The figure shows three views and two pictorial views of one solid part (mm, origin at its lowest corner). Answer the questions. Give positions to 0.01 mm unless a question says otherwise; leave off trailing zeros. Order: outer loops, then holes, each group sorted by start corner. A loop starts at its lowest first (then second) coordinate and runs counter-clockwise, first axis right, second up. Notation, with made-up numbers: (41, 51) - (88, 51) arc R12 ccw to (88, 67) - close; hole circle Ø2 at (62.25, -32). An arc over 180 degrees is marked (long way). Write item = value, one per line.
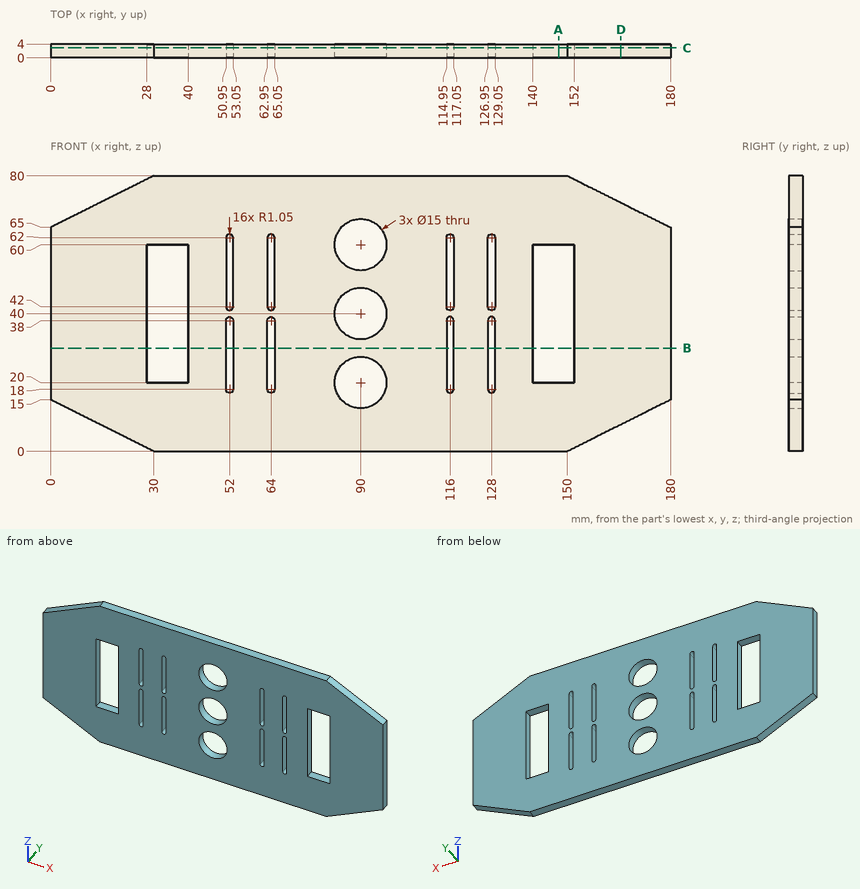
1. Section C-C (y = 2.85) is taken. Count the separate pieces of the cut face and the enclosed holes in it, and give its area (3 significant figures).
Recorded:
separate_pieces = 1
enclosed_holes = 13
area = 11,600 mm^2
2. Straight lines are drawn through the part: L1, parallel to X at y = 1.2, z = 40; L2, parallel to Z at x = 90, y = 1.85; L3, parallel to X at y = 1.35, z = 61.5. For each, find the intervals that lie inside material, in ascending order. Write a range as [from, to].
Recorded:
L1 = [0, 28], [40, 82.5], [97.5, 140], [152, 180]
L2 = [0, 12.5], [27.5, 32.5], [47.5, 52.5], [67.5, 80]
L3 = [0, 50.95], [53.05, 62.95], [65.05, 82.65], [97.35, 114.95], [117.05, 126.95], [129.05, 180]
3. Section B-B (z = 30) is taken. Determine the outline of the cut face in (x, y).
Recorded:
outline = (0, 0) - (28, 0) - (28, 4) - (0, 4) - close; (40, 0) - (50.95, 0) - (50.95, 4) - (40, 4) - close; (53.05, 0) - (62.95, 0) - (62.95, 4) - (53.05, 4) - close; (65.05, 0) - (114.95, 0) - (114.95, 4) - (65.05, 4) - close; (117.05, 0) - (126.95, 0) - (126.95, 4) - (117.05, 4) - close; (129.05, 0) - (140, 0) - (140, 4) - (129.05, 4) - close; (152, 0) - (180, 0) - (180, 4) - (152, 4) - close
4. Section A-A (x = 147.5) is taken. Determine the outline of the cut face in (y, z), and give its area (3 significant figures).
Recorded:
outline = (0, 0) - (4, 0) - (4, 20) - (0, 20) - close; (0, 60) - (4, 60) - (4, 80) - (0, 80) - close
area = 160 mm^2
5. Section D-D (x = 165.5) is taken. Determine the outline of the cut face in (y, z).
Recorded:
outline = (0, 7.75) - (4, 7.75) - (4, 72.25) - (0, 72.25) - close
